from build123d import *

# Parameters (mm, degrees)
F1_DEPTH = 15
F2_R     = 0.49999


# Not quite as in the source:
# - a fillet or chamfer is up to 0.001 mm smaller than in the source, because OpenCascade refuses the exact size


with BuildPart() as f1:
    # F0 (on Top) → F1 (new body)
    with BuildSketch(Plane.XY):
        with BuildLine():
            Line((-5, -12.237534521), (-2, -12.237534521))
            ThreePointArc((-2, -12.237534521), (-1, -11.237534521), (-2, -10.237534521))
            Line((-2, -10.237534521), (-2, 7.762465479))
            ThreePointArc((-2, 7.762465479), (-1.5811388301, 8.9872103504), (-0.5, 9.6989571521))
            Line((-0.5, 9.6989571521), (-0.5, 13.1989571521))
            Line((-0.5, 13.1989571521), (0.5, 13.1989571521))
            Line((0.5, 13.1989571521), (0.5, 9.6989571521))
            ThreePointArc((0.5, 9.6989571521), (1.5811388301, 8.9872103504), (2, 7.762465479))
            Line((2, 7.762465479), (2, -10.237534521))
            ThreePointArc((2, -10.237534521), (1, -11.237534521), (2, -12.237534521))
            Line((2, -12.237534521), (5, -12.237534521))
            Line((5, -12.237534521), (5, 10.762465479))
            ThreePointArc((5, 10.762465479), (0, 15.762465479), (-5, 10.762465479))
            Line((-5, 10.762465479), (-5, -12.237534521))
        make_face()
    extrude(amount=F1_DEPTH)

    # F2 (radius 0.5 in the source; OpenCascade refuses exactly that, so slightly less here)
    f2_edges = [f1.edges().sort_by_distance(p)[0] for p in [
        (-0.5, 13.198957, 7.5),
        (0.5, 13.198957, 7.5),
    ]]
    fillet(f2_edges, radius=F2_R)


solid = f1.part
Geometry check sheet. Reference: the model listing, model coordinates, mm. A direction names the side the tool comes from. Give positions to 0.01 mm unless a question says otherwise; leave off trailing zeros. Loops run counter-clockwise (first coordinate to the right, second up) from the corner with the lowest first, then second, coordinate; pieces in that order, holes last. Notation, with made-up numbers: (-9.75, 51.5) -> (4.25, 51.5) arc R19 ccw to (4.25, 71.5) -> close; hole circle Ø7 at (87, 6). An arc over 180 degrees is marked (long way). Answer in a Markdown table with one row per item. Add a question column.
1) Cross-section at D-D on y = 14.25. Record the boundary of the cut face in (x, z).
2) Draft check along Y on faces 1 (the face through (-5, -1, 7)), 2 (the face through (-2, -1, 7)), 3 (the face through (-4, -12.238, 7)). Enter one of: pulls with the +Y half, pulls with the -Y half, needs draft (parallel to the pull), parting line crosses it, or undercut.
3) Set-up check for faces 4 (the face through (5, -1, 7)), 5 (the face through (1.57, 9, 7.4)), 6 (the face through (-0.5, 11, 7)): record each of +Z, -Z, +X, -X, +Y, -Y from which the full face is reachable in a straight line by a thin tool's end or side.
4) Cross-section at C-C on x = -4. Record the boundary of the cut face in (y, z), and give its area (3 significant figures).
5) Material ranges on probe 1 along X at (y, z) = (4.75, 9.75); probe 2 along X at (y, z) = (10.5, 4); probe 3 along Y at (x, z) = (0, 11), recorded low to high. Write a range as from..to.
6) Cross-section at A-A on y = 2.5. Record the boundary of the cut face in (x, z), and give its area (3 significant figures).
Outcome:
| question | item | result |
|---|---|---|
| 1 | outline | (-3.58, 0) -> (3.58, 0) -> (3.58, 15) -> (-3.58, 15) -> close |
| 2 | face 1 | needs draft |
| 2 | face 2 | undercut |
| 2 | face 3 | pulls with the -Y half |
| 3 | face 4 | +Z, -Z, +X, +Y, -Y |
| 3 | face 5 | +Z, -Z |
| 3 | face 6 | +Z, -Z, -Y |
| 4 | outline | (-12.24, 0) -> (13.76, 0) -> (13.76, 15) -> (-12.24, 15) -> close |
| 4 | area | 390 mm^2 |
| 5 | probe 1 | x = -5..-2, 2..5 |
| 5 | probe 2 | x = -5..-0.5, 0.5..5 |
| 5 | probe 3 | y = 13.2..15.76 |
| 6 | outline | (-5, 0) -> (-2, 0) -> (-2, 15) -> (-5, 15) -> close; (2, 0) -> (5, 0) -> (5, 15) -> (2, 15) -> close |
| 6 | area | 90.0 mm^2 |
